from build123d import *

# Parameters (mm, degrees)
SKETCH1_W           = 144.78
SKETCH1_H           = 233.68
BOSS_EXTRUDE1_DEPTH = 50.8
SKETCH2_W           = 109.22
SKETCH2_H           = 182.88
CUT_EXTRUDE1_DEPTH  = 48.26
CUT_EXTRUDE3_REACH  = 194.856
SKETCH6_W           = 12.7
SKETCH6_H           = 6.85


with BuildPart() as part:
    # Sketch1 → Boss-Extrude1 (new body)
    with BuildSketch(Plane.XY):
        Rectangle(SKETCH1_W, SKETCH1_H)
    extrude(amount=BOSS_EXTRUDE1_DEPTH)

    # Sketch2 → Cut-Extrude1 (cut)
    with BuildSketch(Plane.XY.offset(50.8)):
        Rectangle(SKETCH2_W, SKETCH2_H)
    extrude(amount=-CUT_EXTRUDE1_DEPTH, mode=Mode.SUBTRACT)

    # Sketch6 → Cut-Extrude3 (cut, up to next)
    with BuildSketch(Plane(origin=(72.39, 0, 0), x_dir=(0, 0, -1), z_dir=(1, 0, 0)), mode=Mode.PRIVATE) as cut_extrude3_sk1:
        with Locations((-29.35, 46.215)):
            Rectangle(SKETCH6_W, SKETCH6_H)
    cut_extrude3_tool1 = extrude(cut_extrude3_sk1.sketch, amount=-CUT_EXTRUDE3_REACH, mode=Mode.PRIVATE) & part.part
    # Sketch6 → Cut-Extrude3 (cut, up to next)
    with BuildSketch(Plane(origin=(72.39, 0, 0), x_dir=(0, 0, -1), z_dir=(1, 0, 0)), mode=Mode.PRIVATE) as cut_extrude3_sk2:
        with Locations((-29.35, -73.415)):
            Rectangle(SKETCH6_W, SKETCH6_H)
    cut_extrude3_tool2 = extrude(cut_extrude3_sk2.sketch, amount=-CUT_EXTRUDE3_REACH, mode=Mode.PRIVATE) & part.part
    add(cut_extrude3_tool1.solids().sort_by_distance((72.39, 46.215, 29.35))[0], mode=Mode.SUBTRACT)
    add(cut_extrude3_tool2.solids().sort_by_distance((72.39, -73.415, 29.35))[0], mode=Mode.SUBTRACT)


solid = part.part
Design review of the part built by this model. Coordinates are the model's own, in mm. A direction names the side the tool comes from. Give positions to 0.01 mm unless a question says otherwise; leave off trailing zeros. Loops run counter-clockwise (first coordinate to the right, second up) from the corner with the lowest first, then second, coordinate; pieces in that order, holes last. Notation, with made-up numbers: M 73,45 L 132,45 A16 ccw 132,75 Z; hole C 38.25,89.5 d9. An arc over 180 degrees is marked long. Answer as a JSON object with one key per item and string values.
Item 1: We need section B-B (x = -36). State the section outline as (y, z) points.
Output values:
{"outline": "M -116.84,0 L 116.84,0 L 116.84,50.8 L 91.44,50.8 L 91.44,2.54 L -91.44,2.54 L -91.44,50.8 L -116.84,50.8 Z"}
Item 2: We need section C-C (y = 9.5). State the section outline as (x, z) points, and give its area (3 significant figures).
Output values:
{"outline": "M -72.39,0 L 72.39,0 L 72.39,50.8 L 54.61,50.8 L 54.61,2.54 L -54.61,2.54 L -54.61,50.8 L -72.39,50.8 Z", "area": "2,080 mm2"}
Item 3: We need section D-D (z = 43). State the section outline as (x, y) points, and give its area (3 significant figures).
Output values:
{"outline": "M -72.39,-116.84 L 72.39,-116.84 L 72.39,116.84 L -72.39,116.84 Z; hole M -54.61,-91.44 L 54.61,-91.44 L 54.61,91.44 L -54.61,91.44 Z", "area": "13,900 mm2"}
Item 4: Machinability: for faces 5 (the face through (72.39, -2, 25)), 6 (the face through (64, 46, 35.7)), 7 (the face through (-54.61, -1, 27)), which of the approach directions +Z, -Z, +X, -X, +Y, -Y give a long, thin tool a straight path to every point of the face, cutting with its end or side? Answer none if there is none.
Output values:
{"face 5": "+Z, -Z, +X, +Y, -Y", "face 6": "+X", "face 7": "+Z"}
Item 5: We need section A-A (z = 28.5). State the section outline as (x, y) points.
Output values:
{"outline": "M -72.39,-116.84 L 72.39,-116.84 L 72.39,-76.84 L 54.61,-76.84 L 54.61,-91.44 L -54.61,-91.44 L -54.61,91.44 L 54.61,91.44 L 54.61,49.64 L 72.39,49.64 L 72.39,116.84 L -72.39,116.84 Z; M 54.61,-69.99 L 72.39,-69.99 L 72.39,42.79 L 54.61,42.79 Z"}
Item 6: For P1, Ø6, axis at x = 5.5, y = 22.5, coming from the +Z side, flat-tipped, find the tip position at first contact; note if it passes through.
Output values:
{"P1": "stops at z = 2.54"}
Item 7: Wall thickness on line 1 along X through (y, z) = (-30, 28.5); line 2 along Y through (x, z) = (-47.5, 23.5); line 3 along Z through (x, y) = (54.5, 2.5): over which ranges is each line inside the solid? List them lowest first.
Output values:
{"line 1": "x = -72.39 to -54.61, 54.61 to 72.39", "line 2": "y = -116.84 to -91.44, 91.44 to 116.84", "line 3": "z = 0 to 2.54"}
Item 8: Mouldability with a two-part tool opening along Z and no side actions: class faces 1 (the face through (-1, -116.84, 25)), 2 (the face through (64, -73, 23)), 3 (the face through (-1, 1, 2.54)), 4 (the face through (64, 49.64, 29)) as pulls with the +Z half, pulls with the -Z half, needs draft (parallel to the pull), parting line crosses it, or undercut.
Output values:
{"face 1": "needs draft", "face 2": "undercut", "face 3": "pulls with the +Z half", "face 4": "undercut"}
